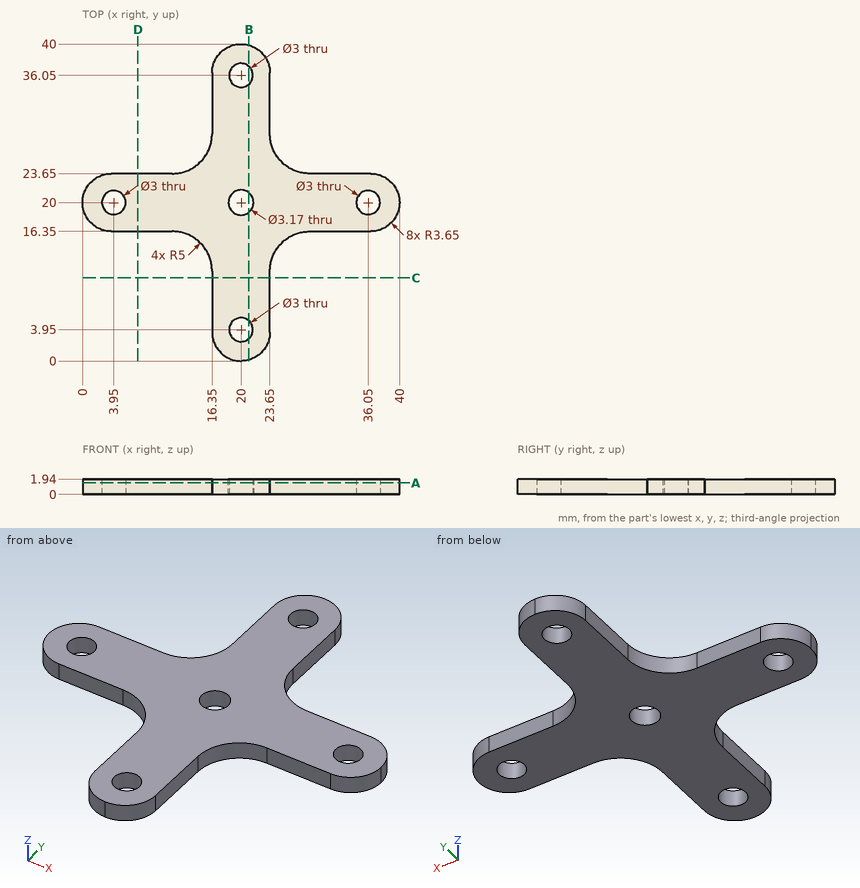
Study the drawing (mm; zero at the part's minimum x, y, z) and answer. Round coordinates to 2 decimals unless told otherwise and drop trailing zeros. Write each loop counter-clockwise with the first axis right and the second up, starting at its lowest first coordinate (ties: lowest second). Pieces come first, ordered by that corner, then holes.
1) Given pin 1 Ø5 at (x, y) = (20, 3.95) entering from -Z; pin 2 Ø0.6 at (y, z) = (6.5, 1) entering from +X; pin 3 Ø0.6 at (x, z) = (32.5, 1) entering from -Y; pin 4 Ø1 at (y, z) = (33.5, 0.5) entering from -X, each flat-ended and moving along its own axis, determine where each tip first touches the part or whether it passes through.
2) A cutting plane is placed at B-B (x = 21). Give the vertices of the cut face in (y, z).
3) Straight lines are drawn through the part: line 1 (Y direction, x = 20, z = 0.65) (3 decimals); line 2 (X direction, y = 36, z = 0.8); line 3 (Y direction, x = 19, z = 1.4). For each, find the intervals that lie inside material, in ascending order.
4) A cutting plane is placed at A-A (z = 1.45). Give the number of separate pieces and of enclosed holes in the cut face, plus the area to 3 significant figures.
5) A cutting plane is placed at C-C (y = 10.5). Give the vertices of the cut face in (x, z), plus the area to 3 significant figures.
Completed:
1. pin 1: stops at z = 0
1. pin 2: stops at x = 23.65
1. pin 3: stops at y = 16.35
1. pin 4: stops at x = 16.35
2. outline: (0.14, 0) - (2.83, 0) - (2.83, 1.94) - (0.14, 1.94) - close; (5.07, 0) - (18.77, 0) - (18.77, 1.94) - (5.07, 1.94) - close; (21.23, 0) - (34.93, 0) - (34.93, 1.94) - (21.23, 1.94) - close; (37.17, 0) - (39.86, 0) - (39.86, 1.94) - (37.17, 1.94) - close
3. line 1: y = 0 to 2.45, 5.45 to 18.415, 21.585 to 34.55, 37.55 to 40
3. line 2: x = 16.35 to 18.5, 21.5 to 23.65
3. line 3: y = 0.14 to 2.83, 5.07 to 18.77, 21.23 to 34.93, 37.17 to 39.86
4. separate pieces: 1
4. enclosed holes: 5
4. area: 493 mm2
5. outline: (16.35, 0) - (23.65, 0) - (23.65, 1.94) - (16.35, 1.94) - close
5. area: 14.2 mm2
